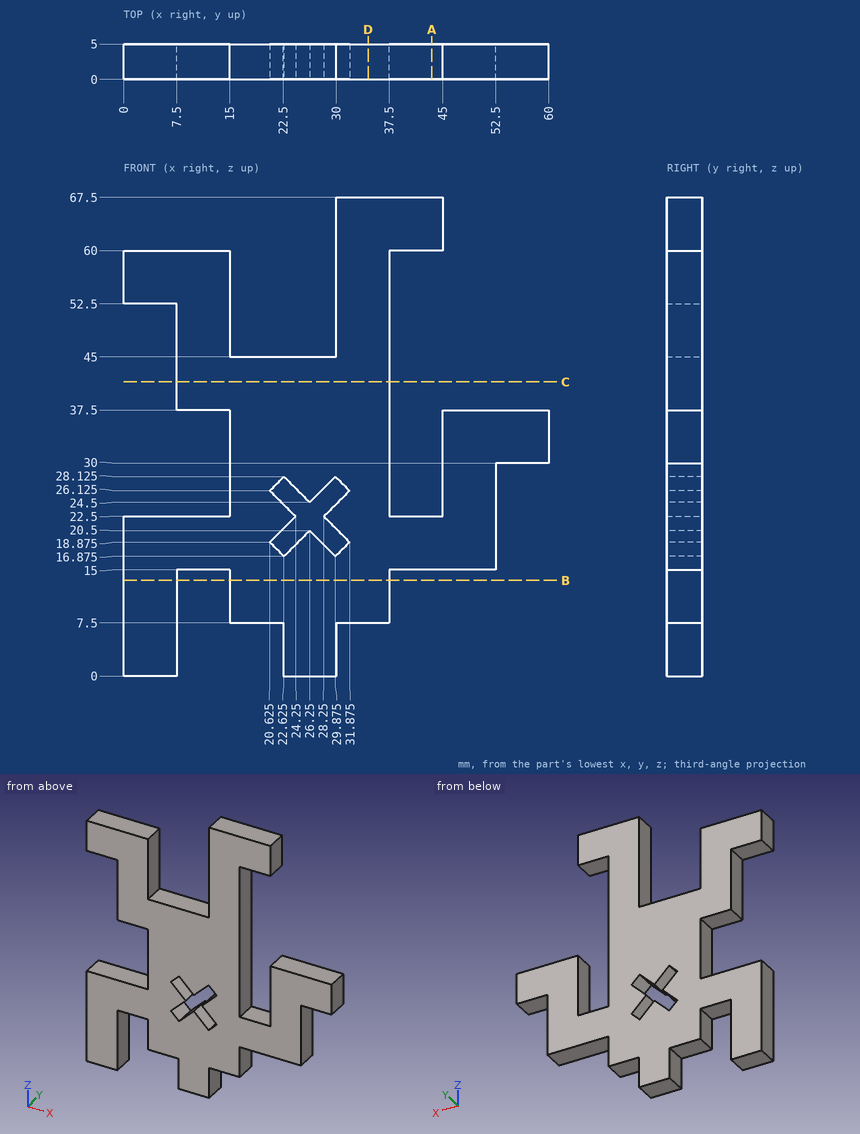
Design review of the part shown in the three views and the two pictorial views. Dimensions are in mm from the part's minimum x, y and z. Round coordinates to 2 decimals unless told otherwise and drop trailing zeros. Loops run counter-clockwise (first coordinate to the right, second up) from the corner with the lowest first, then second, coordinate; pieces in that order, holes last.
Q1. Add section B-B on z = 13.5. Write out the cut boundary in (x, y).
Result sheet:
outline: (0, 0) - (7.5, 0) - (7.5, 5) - (0, 5) - close; (15, 0) - (37.5, 0) - (37.5, 5) - (15, 5) - close
Q2. Insertion check: pin 1 Ø1.5 at (x, y) = (55.5, 3) entering from -Z; pin 2 Ø1 at (y, z) = (3, 19.5) entering from +X; pin 3 Ø2.5 at (y, z) = (3, 13) entering from +X. Each pin has a flat end and moves straight along its axis. Give the tip position at first contact, or say it passes through.
Result sheet:
pin 1: stops at z = 30
pin 2: stops at x = 52.5
pin 3: stops at x = 37.5
Q3. Add section D-D on x = 34.5. Write out the cut boundary in (y, z), plus the area to 3 significant figures.
Result sheet:
outline: (0, 7.5) - (5, 7.5) - (5, 67.5) - (0, 67.5) - close
area: 300 mm2
Q4. To check wall thickness, follow line 1 along X through (y, z) = (4.6, 27); line 2 along X through (y, z) = (1, 33); line 3 along Z through (x, y) = (29, 3.85). State the ranges of each line that lie inside material, in increasing order.
Result sheet:
line 1: x = 15 to 21.5, 23.75 to 28.75, 31 to 37.5, 45 to 52.5
line 2: x = 15 to 37.5, 45 to 60
line 3: z = 0 to 17.75, 21.75 to 23.25, 27.25 to 45
Q5. Add section A-A on x = 43.5. Write out the cut boundary in (y, z).
Result sheet:
outline: (0, 15) - (5, 15) - (5, 22.5) - (0, 22.5) - close; (0, 60) - (5, 60) - (5, 67.5) - (0, 67.5) - close
Q6. Add section C-C on z = 41.5. Write out the cut boundary in (x, y).
Result sheet:
outline: (7.5, 0) - (37.5, 0) - (37.5, 5) - (7.5, 5) - close
